```python
from build123d import *

# Parameters (mm, degrees)
F0_R        = 0.9849519721
F1_DEPTH    = 10
F2_T        = 5
F2_T3_DEPTH = 20
F3_SIZE     = 5
F5_DEPTH    = 25


# Not quite as in the source:
# - a shell that OpenCascade refuses in one call is made with other operations: the cavity is built on its own and cut out


with BuildPart() as f1:
    # F0 (on Front) → F1 (new body)
    with BuildSketch(Plane.XZ):
        with BuildLine():
            Line((25.823418051, 0), (0, 0))
            Line((0, 0), (-25.823418051, 0))
            Line((-25.823418051, 0), (-25.823418051, 7.5157736428))
            Line((-25.823418051, 7.5157736428), (-31.6047780216, 7.5157736428))
            Line((-31.6047780216, 7.5157736428), (-31.6047780216, 0))
            Line((-31.6047780216, 0), (-48.1885363162, 0))
            ThreePointArc((-48.1885363162, 0), (-51.7240702221, -1.4644660941), (-53.1885363162, -5))
            Line((-53.1885363162, -5), (-53.1885363162, -34.1205511987))
            ThreePointArc((-53.1885363162, -34.1205511987), (-51.7240702221, -37.6560851047), (-48.1885363162, -39.1205511987))
            Line((-48.1885363162, -39.1205511987), (0, -39.1205511987))
            Line((0, -39.1205511987), (48.1885363162, -39.1205511987))
            ThreePointArc((48.1885363162, -39.1205511987), (51.7240702221, -37.6560851047), (53.1885363162, -34.1205511987))
            Line((53.1885363162, -34.1205511987), (53.1885363162, -5))
            ThreePointArc((53.1885363162, -5), (51.7240702221, -1.4644660941), (48.1885363162, 0))
            Line((48.1885363162, 0), (31.6047780216, 0))
            Line((31.6047780216, 0), (31.6047780216, 7.5157736428))
            Line((31.6047780216, 7.5157736428), (25.823418051, 7.5157736428))
            Line((25.823418051, 7.5157736428), (25.823418051, 0))
        make_face()
        with Locations((21.3635135442, -24.997510016)):
            Circle(F0_R, mode=Mode.SUBTRACT)
    extrude(amount=F1_DEPTH)

    # F2: shell of thickness 5, made by hand


with BuildPart() as f2_core1:
    # F2_t2: copy of F1
    add(f1.part)

    # the walls: a layer under each face that stays
    f2_faces = [f2_core1.faces().sort_by_distance(p)[0] for p in [
        (39.8966571689, -5, 0),
        (20.3785615721, -5, -24.997510016),
        (53.1885363162, -5, -19.5602755994),
        (0, -5, -39.1205511987),
        (-53.1885363162, -5, -19.5602755994),
        (-39.8966571689, -5, 0),
        (-31.6047780216, -5, 3.7578868214),
        (-28.7140980363, -5, 7.5157736428),
        (-25.823418051, -5, 3.7578868214),
        (0, -5, 0),
        (25.823418051, -5, 3.7578868214),
        (28.7140980363, -5, 7.5157736428),
        (0, 0, -15.802388778),
        (31.6047780216, -5, 3.7578868214),
    ]]
    thicken(f2_faces, amount=-F2_T, mode=Mode.SUBTRACT)

    # F2_s4 → F2_t3 (cut)
    with BuildSketch(Plane.XZ.offset(-5)):
        Polygon((31.6547780216, 0.05), (31.6047780216, -5), (26.6047780216, -5), (26.6047780216, 0), align=None)
        Polygon((-31.6547780216, 0.05), (-31.6047780216, -5), (-26.6047780216, -5), (-26.6047780216, 0), align=None)
        Polygon((-25.773418051, 0.05), (-30.823418051, 0), (-30.823418051, -5), (-25.823418051, -5), align=None)
        Polygon((25.773418051, 0.05), (25.823418051, -5), (30.823418051, -5), (30.823418051, 0), align=None)
    extrude(amount=F2_T3_DEPTH, mode=Mode.SUBTRACT)


with BuildPart() as f1_1:
    add(f1.part)

    # what is left inside the walls is the cavity
    f2_cavity = [f2_core1.part.solids().sort_by_distance(p)[0] for p in [
        (0, -9.95, -24.413701),
    ]]
    add(f2_cavity, mode=Mode.SUBTRACT)

    # F3
    f3_edges = [f1_1.edges().sort_by_distance(p)[0] for p in [
        (-31.604778, -5, 7.515774),
        (31.604778, -5, 7.515774),
    ]]
    chamfer(f3_edges, length=F3_SIZE)

    # F4 (on face) → F5 (cut)
    with BuildSketch(Plane(origin=(0, 0, 0), x_dir=(-1, 0, 0), z_dir=(0, 1, 0))):
        with BuildLine():
            Line((21.4935876429, -36.0602382571), (21.4935876429, -9.7583141178))
            Line((21.4935876429, -9.7583141178), (-21.4935876429, -9.7583141178))
            Line((-21.4935876429, -9.7583141178), (-21.4935876429, -24.0211847033))
            ThreePointArc((-21.4935876429, -24.0211847033), (-20.714663158, -24.2564812961), (-20.3785615721, -24.997510016))
            ThreePointArc((-20.3785615721, -24.997510016), (-20.714663158, -25.7385387358), (-21.4935876429, -25.9738353286))
            Line((-21.4935876429, -25.9738353286), (-21.4935876429, -36.0602382571))
            Line((-21.4935876429, -36.0602382571), (21.4935876429, -36.0602382571))
        make_face()
    extrude(amount=-F5_DEPTH, mode=Mode.SUBTRACT)


solid = f1_1.part
```
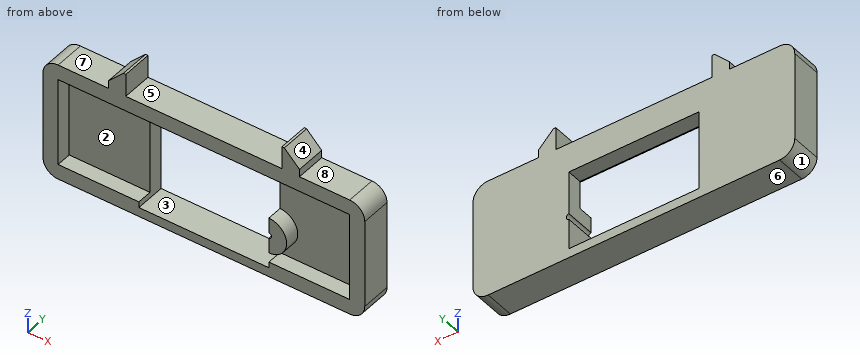
Design review of the part built by this model. Coordinates are the model's own, in mm. Face numbers are marked on the shaded views. A direction names the side the tool comes from. Give positions to 0.01 mm unless a question says otherwise; leave off trailing zeros. Loops run counter-clockwise (first coordinate to the right, second up) from the corner with the lowest first, then second, coordinate; pieces in that order, holes last. Notation, with made-up numbers: M 16,36.5 L 65,36.5 A36 cw 65,71.5 Z; hole C 50,64 d10. An arc over 180 degrees is marked long. Return JSON: item names as keys, results as strings. Group by question number.
Item 1: Tool access review of the marked faces 5, 6, 7 and 8: name each direction out of +Z, -Z, +X, -X, +Y, -Y from which nothing blocks a thin tool from reaching the whole face with its end or side.
Item 2: We need section A-A (y = -7.5). Give the number of separate pieces and of enclosed holes in the cut face, and give its area (3 significant figures).
Item 3: Mouldability with a two-part tool opening along Z and no side actions: class the marked faces 1, 2, 3 and 4 as released by +Z, released by -Z, zero draft, split by the parting line, or undercut.
Item 4: Insertion check: pin 1 Ø4 at (x, y) = (-37, -8.5) entering from +Z; pin 2 Ø4 at (y, z) = (-4.5, 4) entering from -X; pin 3 Ø3 at (x, z) = (-34.5, -25.5) entering from -Y. Each pin has a flat end and moves straight along its axis. Give the tip position at first contact, or say it passes through.
Item 5: We need section D-D (z = -16). Give the boundary of the cut face in (x, y).
Item 6: For probe 1 along X at (y, z) = (-6.75, -25); probe 2 along X at (y, z) = (-3, -27.5); probe 3 along Z at (x, y) = (-7, -8.5), list the stretches that pass through material, from the lowest coordinate up.
Item 7: We need section C-C (y = -2). Give the boundary of the cut face in (x, z).
Item 8: We need section B-B (x = 2). Give the boundary of the cut face in (y, z), and give its area (3 significant figures).
Output:
{
 "1": {"face 5": "+Z, +Y, -Y", "face 6": "-Z, +X, -X, +Y, -Y", "face 7": "+Z, -X, +Y, -Y", "face 8": "+Z, +X, +Y, -Y"},
 "2": {"separate pieces": "2", "enclosed holes": "1", "area": "1,370 mm^2"},
 "3": {"face 1": "released by -Z", "face 2": "undercut", "face 3": "undercut", "face 4": "released by +Z"},
 "4": {"pin 1": "stops at z = 0", "pin 2": "stops at x = -31.6", "pin 3": "stops at y = -5"},
 "5": {"outline": "M -53.19,-10 L -48.19,-10 L -48.19,-5 L -21.49,-5 L -21.49,0 L -53.19,0 Z; M 21.49,-5 L 48.19,-5 L 48.19,-10 L 53.19,-10 L 53.19,0 L 21.49,0 Z"},
 "6": {"probe 1": "x = -53.19 to -48.19, 22.35 to 27.35, 48.19 to 53.19", "probe 2": "x = -53.19 to -21.49, 21.49 to 53.19", "probe 3": "z = -39.12 to -36.06, -5 to 0"},
 "7": {"outline": "M -53.19,-34.12 A5 ccw -48.19,-39.12 L 48.19,-39.12 A5 ccw 53.19,-34.12 L 53.19,-5 A5 ccw 48.19,0 L 31.6,0 L 31.6,2.52 L 26.6,7.52 L 25.82,7.52 L 25.82,0 L -25.82,0 L -25.82,7.52 L -26.6,7.52 L -31.6,2.52 L -31.6,0 L -48.19,0 A5 ccw -53.19,-5 Z; hole M -21.49,-36.06 L 21.49,-36.06 L 21.49,-25.97 A0.98 ccw 21.49,-24.02 L 21.49,-9.76 L -21.49,-9.76 Z"},
 "8": {"outline": "M -10,-39.12 L 0,-39.12 L 0,-36.06 L -10,-36.06 Z; M -10,-5 L -5,-5 L -5,-9.76 L 0,-9.76 L 0,0 L -10,0 Z", "area": "104 mm^2"}
}
